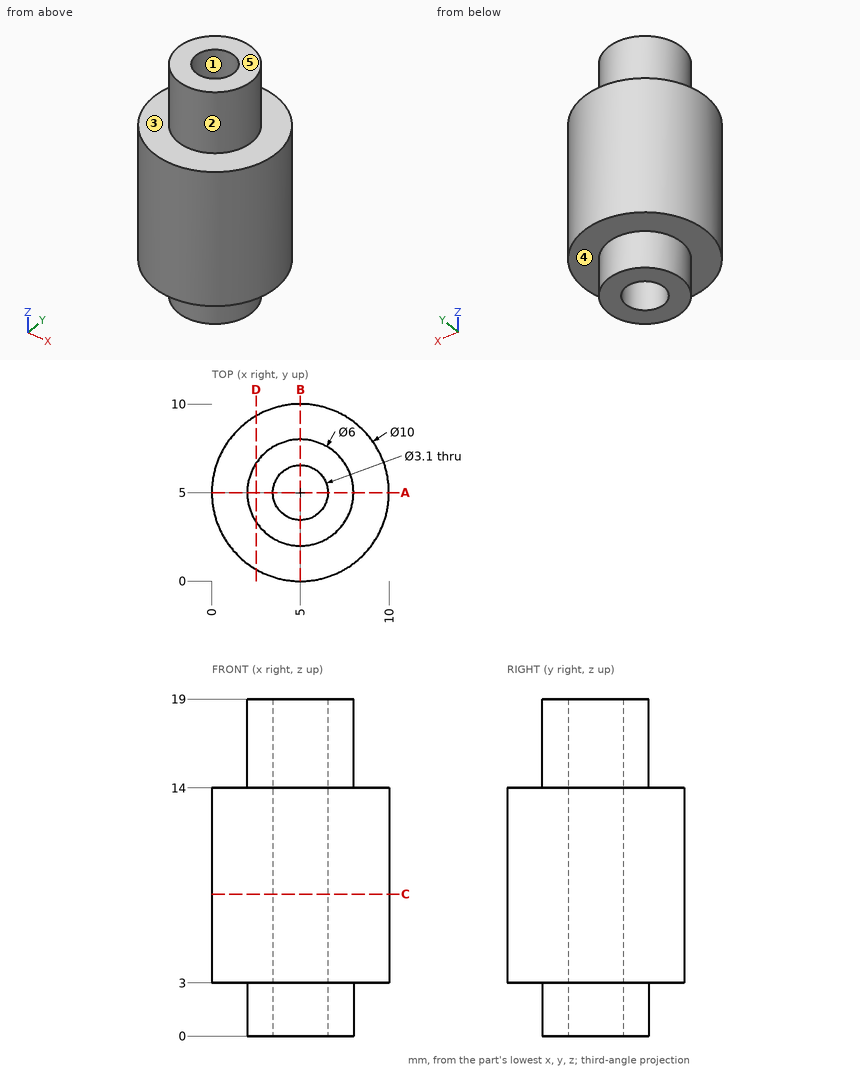
Geometry check sheet. Reference: drawing and pictorial views, mm from the part's lowest x, y, z. A direction names the side the tool comes from. Coordinates: 2 decimals unless noted, no trailing zeros. Loops run counter-clockwise (first coordinate to the right, second up) from the corner with the lowest first, then second, coordinate; pieces in that order, holes last. Notation, with made-up numbers: M 11,28 L 37,28 A28 ccw 37,54 Z; hole C 84,5.25 d1. An arc over 180 degrees is marked long. One line per item, written item: value.
1. Set-up check for the marked faces 4 and 5: record each of +Z, -Z, +X, -X, +Y, -Y from which the full face is reachable in a straight line by a thin tool's end or side.
Answers follow:
face 4: -Z
face 5: +Z, +X, -X, +Y, -Y
2. Section check A-A on y = 5. Record the cut outline in (x, z), plus the area to 3 significant figures.
Answers follow:
outline: M 0,3 L 2,3 L 2,0 L 3.45,0 L 3.45,19 L 2,19 L 2,14 L 0,14 Z; M 6.55,0 L 8,0 L 8,3 L 10,3 L 10,14 L 8,14 L 8,19 L 6.55,19 Z
area: 99.1 mm^2
3. Gauge pin test, flat ends, axial feed: P1, Ø3, axis at y = 2, z = 13.5, coming from the +X side; P2, Ø2, axis at x = 8.5, z = 3, coming from the +Y side; P3, Ø2, axis at x = 1.5, z = 5.5, coming from the -Y side; P4, Ø3, axis at x = 5, y = 5, coming from the -Z side. Record the tip position at first contact, or that the pin passes through.
Answers follow:
P1: x = 9.77
P2: y = 9.33
P3: y = 0.67
P4: through
4. Section check C-C on z = 8. Record the cut outline in (x, y).
Answers follow:
outline: C 5,5 d10; hole C 5,5 d3.1
5. Material ranges on line 1 along Y through (x, z) = (5, 14.5); line 2 along Y through (x, z) = (5, 12), recorded low to high. Write a range as from..to.
Answers follow:
line 1: 2..3.45, 6.55..8
line 2: 0..3.45, 6.55..10
6. Section check D-D on x = 2.5. Record the cut outline in (y, z).
Answers follow:
outline: M 0.67,3 L 3.34,3 L 3.34,0 L 6.66,0 L 6.66,3 L 9.33,3 L 9.33,14 L 6.66,14 L 6.66,19 L 3.34,19 L 3.34,14 L 0.67,14 Z
7. Mould release check, pull along X, two halves, no side actions. Record for the marked faces 1, 2 and 3: pulls with the +X half, pulls with the -X half, needs draft (parallel to the pull), parting line crosses it, or undercut.
Answers follow:
face 1: undercut
face 2: parting line crosses it
face 3: needs draft
